Check sheet for the modelled part. Datum: model origin and axes. Units: mm. A direction names the side the tool comes from. Round coordinates to 2 decimals unless told otherwise and drop trailing zeros. Order: outer loops, then holes, each group sorted by start corner. A loop starts at its lowest first (then second) coordinate and runs counter-clockwise, first axis right, second up. Notation, with made-up numbers: (17.5, 22.25) -> (29.5, 22.25) arc R23 cw to (29.5, 42.25) -> close; hole circle Ø9 at (86, 26). An arc over 180 degrees is marked (long way). Use CSV: the item, a comma, the result in double quotes.
```python
from build123d import *

# Parameters (mm, degrees)
F0_R     = 3.96875
F1_DEPTH = 9.525
F2_R     = 3.175
F3_DEPTH = 3.175
F4_R     = 3.96875
F5_DEPTH = 9.525
F6_R     = 3.175
F7_DEPTH = 3.175
F8_SIZE  = 0.254


with BuildPart() as f1:
    # F0 (on Top) → F1 (new body)
    with BuildSketch(Plane.XY):
        Circle(F0_R)
    extrude(amount=F1_DEPTH)



with BuildPart() as f3:
    # F2 (on face) → F3 (new body)
    with BuildSketch(Plane(origin=(0, 0, -9.525), x_dir=(1, 0, 0), z_dir=(0, 0, -1))):
        Circle(F2_R)
    extrude(amount=F3_DEPTH)


with BuildPart() as f1_1:
    add(f1.part)

    add(f3.part)  # F5 merges F3
    # F4 (on face) → F5 (join)
    with BuildSketch(Plane(origin=(0, 0, 0), x_dir=(1, 0, 0), z_dir=(0, 0, -1))):
        Circle(F4_R)
    extrude(amount=F5_DEPTH)

    # F6 (on face) → F7 (join)
    with BuildSketch(Plane.XY.offset(9.525)):
        Circle(F6_R)
    extrude(amount=F7_DEPTH)

    # F8
    f8_edges = [f1_1.edges().sort_by_distance(p)[0] for p in [
        (-3.175, 0, -12.7),
        (-3.96875, 0, 9.525),
        (-3.96875, 0, -9.525),
        (-3.175, 0, 12.7),
    ]]
    chamfer(f8_edges, length=F8_SIZE)


solid = f1_1.part
```
Q1. Sectioned sample at A-A, the plane x = 0. Enter the section's corners in (y, z) (3 decimals), then the cut area to 3 significant figures.
Result sheet:
outline,"(-3.969, -9.271) -> (-3.715, -9.525) -> (-3.175, -9.525) -> (-3.175, -12.446) -> (-2.921, -12.7) -> (2.921, -12.7) -> (3.175, -12.446) -> (3.175, -9.525) -> (3.715, -9.525) -> (3.969, -9.271) -> (3.969, 9.271) -> (3.715, 9.525) -> (3.175, 9.525) -> (3.175, 12.446) -> (2.921, 12.7) -> (-2.921, 12.7) -> (-3.175, 12.446) -> (-3.175, 9.525) -> (-3.715, 9.525) -> (-3.969, 9.271) -> close"
area,"191 mm^2"
Q2. Scan lines: L1, parallel to Z at x = 2.25, y = 2.5 (3 decimals); L2, parallel to Y at x = 1.5, z = -2.5. Record each from-to range of solid material in increasing order.
Result sheet:
L1,"z = -9.525 to 9.525"
L2,"y = -3.67 to 3.67"
Q3. Sectioned sample at C-C, the plane z = 0.5. Enter the section's corners in (x, y).
Result sheet:
outline,"circle Ø7.94 at (0, 0)"
Q4. Go/stop test with flat-tipped pins: pin 1 (1 mm diameter, centred on x = 0.5, z = 9.5, fed in from +Y); pin 2 (4 mm diameter, centred on x = -2.5, z = -5, fed in from -Y); pin 3 (1.5 mm diameter, centred on y = 3, z = -7, fed in from -X); pin 4 (1 mm diameter, centred on x = -3, y = 3, fed in from -Z). Record where each tip stops, or that it passes through.
Result sheet:
pin 1,"stops at y = 3.97"
pin 2,"stops at y = -3.94"
pin 3,"stops at x = -3.27"
pin 4,"stops at z = -9.5"
Q5. Access from +Z, -Z, +X, -X, +Y, -Y to the whole of each face (thin tool, end or side, straight path). Record for faces 1 (the face through (-0.69, -3.1, 10.97)), 2 (the face through (0, 0, -12.7)), 3 (the face through (-0.69, 3.1, -10.97)).
Result sheet:
face 1,"+Z"
face 2,"-Z, +X, -X, +Y, -Y"
face 3,"-Z"
